The listing builds one solid part. Answer for the finished solid, in the listing's coordinates (mm). Face numbers are marked on the shaded views. A direction names the side the tool comes from. Round coordinates to 2 decimals unless told otherwise and drop trailing zeros. Write each loop counter-clockwise with the first axis right and the second up, starting at its lowest first coordinate (ties: lowest second). Pieces come first, ordered by that corner, then holes. Notation, with made-up numbers: (79, 62) - (98, 62) arc R31 ccw to (98, 93) - close; hole circle Ø9 at (15, -32.75). An arc over 180 degrees is marked (long way). Use a Markdown table: item, result. Add a question column.
1) A cutting plane is placed at C-C (y = 10). Give the vertices of the cut face in (x, z), then the cut area to 3 significant figures.
2) Each of these flat-tipped pins is pushed along its axis until it touches: P1, Ø2, axis at y = 4, z = -25.5, coming from the -X side; P2, Ø10, axis at x = -7.5, y = 16, coming from the -Z side; P3, Ø5, axis at x = -7, z = -26, coming from the +Y side; P4, Ø8, axis at x = 7.5, z = -25, coming from the -Y side. Where does it stop, or does it pass through?
3) A cutting plane is placed at A-A (x = -7.5). Give the vertices of the cut face in (y, z), then the cut area to 3 significant figures.
4) Determine the mould class of the marked faces 1, 2, 3 and 4 for opening direction Y: +Y half, -Y half, draft (parallel to the pull), parting line (faces both ways), or undercut.
5) A cutting plane is placed at B-B (z = -12). Give the vertices of the cut face in (x, y), then the cut area to 3 significant figures.
6) A tool of negligible diameter and unlimited length cuts with its end or side. For the marked faces 5 and 6, from which of +Z, -Z, +X, -X, +Y, -Y can it reach the whole face along a straight path? Write none if from no direction.
7) Find the intervals of material crossed by probe 1 along X at (y, z) = (19.75, 25); probe 2 along Z at (x, y) = (6.25, 19); probe 3 along Y at (x, z) = (5, -3), in increasing order. Write a range as from..to.
8) A cutting plane is placed at D-D (z = 25). Give the vertices of the cut face in (x, y).
```python
from build123d import *

# Parameters (mm, degrees)
SKETCH1_W           = 30
SKETCH1_H           = 80
BOSS_EXTRUDE1_DEPTH = 27
SKETCH2_R           = 5
CUT_EXTRUDE1_DEPTH  = 40
FILLET5_R           = 40
FILLET6_R           = 40
FILLET7_R           = 2
FILLET8_R           = 2
SKETCH6_R           = 5
CUT_EXTRUDE3_DEPTH  = 10


with BuildPart() as part:
    # Sketch1 → Boss-Extrude1 (new body)
    with BuildSketch(Plane(origin=(0, 0, 0), x_dir=(1, 0, 0), z_dir=(0, 1, 0))):
        Rectangle(SKETCH1_W, SKETCH1_H)
    extrude(amount=BOSS_EXTRUDE1_DEPTH)

    # Sketch2 → Cut-Extrude1 (cut)
    with BuildSketch(Plane(origin=(15, 0, 0), x_dir=(0, 0, -1), z_dir=(1, 0, 0))):
        with Locations((-12, 13.5)):
            Circle(SKETCH2_R)
        with Locations(Location((12, 13.5, 0), (0, 0, 180))):
            Circle(SKETCH2_R)
    extrude(amount=-CUT_EXTRUDE1_DEPTH, mode=Mode.SUBTRACT)

    # Fillet5
    # the kernel refuses this fillet: 40 mm, written as the material it takes off along each edge
    with BuildSketch(Plane(origin=(109.571401597, 0, -40), x_dir=(0, 0, 1), z_dir=(-1, 0, 0))) as fillet5_piece_1:
        with BuildLine():
            CenterArc((37.828560639, 40), FILLET5_R, 198.965574989, 71.034425011)
            Line((0, 27), (-0.756571213, 26.74))
            ThreePointArc((-0.756571213, 26.74), (-0.8, 13.5), (-0.8, 0))
            Line((-0.8, 0), (0, -0.8))
            Line((0, -0.8), (37.828560639, -0.8))
            Line((37.828560639, -0.8), (37.828560639, 0))
        make_face()
    extrude(amount=219.142803194, mode=Mode.SUBTRACT)

    # Fillet6
    # the kernel refuses this fillet: 40 mm, written as the material it takes off along each edge
    with BuildSketch(Plane(origin=(-109.571401597, 0, 40), x_dir=(0, 1, 0), z_dir=(1, 0, 0))) as fillet6_piece_1:
        with BuildLine():
            CenterArc((40, -37.828560639), FILLET6_R, 108.965574989, 71.034425011)
            Line((0, -37.828560639), (-0.8, -37.828560639))
            Line((-0.8, -37.828560639), (-0.8, 0))
            Line((-0.8, 0), (0, 0.8))
            ThreePointArc((0, 0.8), (13.5, 0.8), (26.74, 0.756571213))
            Line((26.74, 0.756571213), (27, 0))
        make_face()
    extrude(amount=219.142803194, mode=Mode.SUBTRACT)

    # Fillet7
    fillet7_edges = [part.edges().sort_by_distance(p)[0] for p in [
        (0, 27, -40),
    ]]
    fillet(fillet7_edges, radius=FILLET7_R)

    # Fillet8
    fillet8_edges = [part.edges().sort_by_distance(p)[0] for p in [
        (0, 27, 40),
    ]]
    fillet(fillet8_edges, radius=FILLET8_R)

    # Sketch6 → Cut-Extrude3 (cut)
    with BuildSketch(Plane(origin=(0, 27, 0), x_dir=(1, 0, 0), z_dir=(0, 1, 0))):
        with Locations(Location((-7.5, 25, 0), (0, 0, 270))):
            Circle(SKETCH6_R)
        with Locations(Location((7.5, 25, 0), (0, 0, 270))):
            Circle(SKETCH6_R)
        with Locations(Location((7.5, -25, 0), (0, 0, 90))):
            Circle(SKETCH6_R)
        with Locations(Location((-7.5, -25, 0), (0, 0, 90))):
            Circle(SKETCH6_R)
    extrude(amount=-CUT_EXTRUDE3_DEPTH, mode=Mode.SUBTRACT)


solid = part.part
```
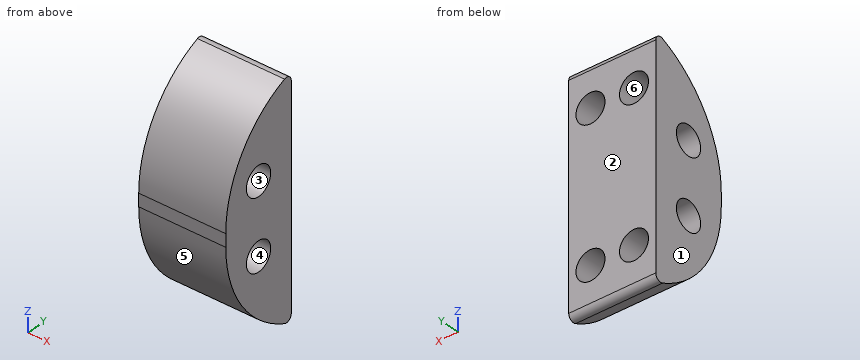
Entries:
| question | item | result |
|---|---|---|
| 1 | outline | (-15, -28.63) - (15, -28.63) - (15, -15.57) - (-15, -15.57) - close; (-15, -8.43) - (15, -8.43) - (15, 8.43) - (-15, 8.43) - close; (-15, 15.57) - (15, 15.57) - (15, 28.63) - (-15, 28.63) - close |
| 1 | area | 1,290 mm² |
| 2 | P1 | passes through |
| 2 | P2 | stops at z = -37.37 |
| 2 | P3 | stops at y = 17 |
| 2 | P4 | stops at y = 4.71 |
| 3 | outline | (0, -2.17) arc R40 ccw to (24.21, -38.92) arc R2 ccw to (27, -37.09) - (27, -30) - (17, -30) - (17, -20) - (27, -20) - (27, 20) - (17, 20) - (17, 30) - (27, 30) - (27, 37.09) arc R2 ccw to (24.21, 38.92) arc R40 ccw to (0, 2.17) - close; hole circle Ø10 at (13.5, -12); hole circle Ø10 at (13.5, 12) |
| 3 | area | 1,250 mm² |
| 4 | face 1 | draft |
| 4 | face 2 | +Y half |
| 4 | face 3 | undercut |
| 4 | face 4 | undercut |
| 5 | outline | (-15, 1.23) - (15, 1.23) - (15, 8.5) - (-15, 8.5) - close; (-15, 18.5) - (15, 18.5) - (15, 27) - (-15, 27) - close |
| 5 | area | 473 mm² |
| 6 | face 5 | -Z, +X, -X, -Y |
| 6 | face 6 | +Y |
| 7 | probe 1 | x = -15..-12.5, -2.5..2.5, 12.5..15 |
| 7 | probe 2 | z = -36.22..-29.84, -20.16..20.16, 29.84..36.22 |
| 7 | probe 3 | y = 0.01..27 |
| 8 | outline | (-15, 7.15) - (15, 7.15) - (15, 27) - (12.5, 27) - (12.5, 17) - (2.5, 17) - (2.5, 27) - (-2.5, 27) - (-2.5, 17) - (-12.5, 17) - (-12.5, 27) - (-15, 27) - close |
